Read the model definition and answer for the solid it produces. Units are mm, in the model's axes. A direction names the side the tool comes from. Round coordinates to 2 decimals unless told otherwise and drop trailing zeros. Loops run counter-clockwise (first coordinate to the right, second up) from the corner with the lowest first, then second, coordinate; pieces in that order, holes last. Notation, with made-up numbers: M 13,-17 L 52,-17 A32 cw 52,19 Z; hole C -11.75,36.5 d9. An arc over 180 degrees is marked long. Write each question's results on one line, items separated by ' | '.
```python
from build123d import *

# Parameters (mm, degrees)
F0_W     = 609.6
F0_H     = 647.7
F1_DEPTH = 314.325
F2_R     = 22.225
F3_DEPTH = 114.3
F4_W     = 609.6
F4_H     = 12.7
F5_DEPTH = 114.3
F6_W     = 609.6
F6_H     = 647.7
F6_W_2   = 603.25
F6_H_2   = 641.35
F7_DEPTH = 15.875


with BuildPart() as f1:
    # F0 (on Front) → F1 (new body, symmetric)
    with BuildSketch(Plane.XZ):
        with Locations((0, 438.15)):
            Rectangle(F0_W, F0_H)
    extrude(amount=F1_DEPTH, both=True)

    # F2 (on Top) → F3 (join)
    with BuildSketch(Plane.XY):
        with Locations((-228.6, -238.125)):
            Circle(F2_R)
        with Locations((228.6, -238.125)):
            Circle(F2_R)
        with Locations((228.6, 238.125)):
            Circle(F2_R)
        with Locations((-228.6, 238.125)):
            Circle(F2_R)
    extrude(amount=F3_DEPTH)

    # F4 (on Top) → F5 (join, through all)
    with BuildSketch(Plane.XY):
        with Locations((0, -266.954)):
            Rectangle(F4_W, F4_H)
    extrude(amount=F5_DEPTH)

    # F6 (on face) → F7 (cut)
    with BuildSketch(Plane.XZ.offset(314.325)):
        with Locations((0, 438.15)):
            Rectangle(F6_W, F6_H)
        with Locations((0, 438.15)):
            Rectangle(F6_W_2, F6_H_2, mode=Mode.SUBTRACT)
    extrude(amount=-F7_DEPTH, mode=Mode.SUBTRACT)


solid = f1.part
```
1. Determine the mould class of faces 1 (the face through (-229, -238, 0)), 2 (the face through (-218.34, 218.41, 56.35)), 3 (the face through (-304.8, 4, 376)), 4 (the face through (-218.34, -257.84, 56.35)) for opening direction X: released by +X, released by -X, zero draft, split by the parting line, or undercut.
Completed:
face 1: zero draft | face 2: undercut | face 3: released by -X | face 4: undercut
2. Find section C-C, the plane y = 55. Give the vertices of the cut face in (x, z).
Completed:
outline: M -304.8,114.3 L 304.8,114.3 L 304.8,762 L -304.8,762 Z
3. Given P1, Ø1, axis at x = 84.5, y = 106.5, coming from the -Z side; P2, Ø5, axis at x = -5, y = -305, coming from the +Z side (3 decimals); P3, Ø5, axis at x = -129, y = -306.5, coming from the -Z side (3 decimals), each flat-ended and moving along its own axis, determine where each tip first touches the part or whether it passes through.
Completed:
P1: stops at z = 114.3 | P2: stops at z = 758.825 | P3: stops at z = 117.475
4. Which of the six approach directions +Z, -Z, +X, -X, +Y, -Y give full straight-line access (tool end or side, diameter ignored) to faces 5 (the face through (-4, -273.304, 56)), 6 (the face through (238.86, 218.41, 56.35)), 7 (the face through (228, 238, 0))?
Completed:
face 5: -Z, +X, -X, -Y | face 6: -Z | face 7: -Z, +X, -X, +Y, -Y
5. Find section A-A, the plane z = 80.5. Give the vertices of the cut face in (x, y) (3 decimals), then the cut area to 3 significant figures.
Completed:
outline: M -304.8,-273.304 L 304.8,-273.304 L 304.8,-260.604 L -304.8,-260.604 Z; C -228.6,-238.125 d44.45; C -228.6,238.125 d44.45; C 228.6,-238.125 d44.45; C 228.6,238.125 d44.45 | area: 13,900 mm2
6. Find section B-B, the plane x = -52. Give the vertices of the cut face in (y, z) (3 decimals).
Completed:
outline: M -314.325,117.475 L -298.45,117.475 L -298.45,114.3 L -273.304,114.3 L -273.304,0 L -260.604,0 L -260.604,114.3 L 314.325,114.3 L 314.325,762 L -298.45,762 L -298.45,758.825 L -314.325,758.825 Z
7. Find section D-D, the plane x = -228.6. Give the vertices of the cut face in (y, z) (3 decimals), then the cut area to 3 significant figures.
Completed:
outline: M -314.325,117.475 L -298.45,117.475 L -298.45,114.3 L -273.304,114.3 L -273.304,0 L -260.604,0 L -260.604,114.3 L -260.35,114.3 L -260.35,0 L -215.9,0 L -215.9,114.3 L 215.9,114.3 L 215.9,0 L 260.35,0 L 260.35,114.3 L 314.325,114.3 L 314.325,762 L -298.45,762 L -298.45,758.825 L -314.325,758.825 Z | area: 419,000 mm2
8. Find the intervals of material crossed by L1, parallel to Z at x = 191.5, y = 63.5; L2, parallel to Y at x = -172, z = 84, in increasing order.
Completed:
L1: z = 114.3 to 762 | L2: y = -273.3 to -260.6
